Design review of the part built by this model. Coordinates are the model's own, in mm. Face numbers are marked on the shaded views. A direction names the side the tool comes from. Give positions to 0.01 mm unless a question says otherwise; leave off trailing zeros. Order: outer loops, then holes, each group sorted by start corner. A loop starts at its lowest first (then second) coordinate and runs counter-clockwise, first axis right, second up. Notation, with made-up numbers: (55, -25) -> (65, -25) arc R28 cw to (65, -6) -> close; hole circle Ø7 at (46, 52.25). An arc over 180 degrees is marked (long way). Return JSON: item names as keys, results as strings.
```python
from build123d import *

# Parameters (mm, degrees)
SKETCH1_R           = 11.1125
BOSS_EXTRUDE1_DEPTH = 29.028571429
SKETCH2_R           = 9.525
BOSS_EXTRUDE2_DEPTH = 44.45
SKETCH3_W           = 2.553411187
SKETCH3_H           = 10.53028371
SKETCH3_W_2         = 2.754606744
CUT_EXTRUDE1_DEPTH  = 44.45
SKETCH4_R           = 6.35
BOSS_EXTRUDE3_DEPTH = 1.5875
SKETCH5_W           = 1.859243387
SKETCH5_H           = 6.148361062
SKETCH5_W_2         = 2.232892279
CUT_EXTRUDE2_DEPTH  = 1.5875
SKETCH6_R           = 2.38125
BOSS_EXTRUDE4_DEPTH = 11.1125


with BuildPart() as part:
    # Sketch1 → Boss-Extrude1 (new body)
    with BuildSketch(Plane(origin=(0, 0, 0), x_dir=(0, 0, -1), z_dir=(1, 0, 0))):
        Circle(SKETCH1_R)
    extrude(amount=BOSS_EXTRUDE1_DEPTH)

    # Sketch2 → Boss-Extrude2 (add)
    with BuildSketch(Plane(origin=(29.028571429, 0, 0), x_dir=(0, 0, -1), z_dir=(1, 0, 0))):
        Circle(SKETCH2_R)
    extrude(amount=BOSS_EXTRUDE2_DEPTH)

    # Sketch3 → Cut-Extrude1 (cut)
    with BuildSketch(Plane(origin=(73.478571429, 0, 0), x_dir=(0, 0, -1), z_dir=(1, 0, 0))):
        with Locations((-9.214205594, 0)):
            Rectangle(SKETCH3_W, SKETCH3_H)
        with Locations((9.314803372, 0)):
            Rectangle(SKETCH3_W_2, SKETCH3_H)
    extrude(amount=-CUT_EXTRUDE1_DEPTH, mode=Mode.SUBTRACT)

    # Sketch4 → Boss-Extrude3 (add)
    with BuildSketch(Plane.ZY):
        Circle(SKETCH4_R)
    extrude(amount=BOSS_EXTRUDE3_DEPTH)

    # Sketch5 → Cut-Extrude2 (cut)
    with BuildSketch(Plane.ZY.offset(1.5875)):
        with Locations((-6.485871694, 0)):
            Rectangle(SKETCH5_W, SKETCH5_H)
        with Locations((6.67269614, 0)):
            Rectangle(SKETCH5_W_2, SKETCH5_H)
    extrude(amount=-CUT_EXTRUDE2_DEPTH, mode=Mode.SUBTRACT)

    # Sketch6 → Boss-Extrude4 (add)
    with BuildSketch(Plane.ZY.offset(1.5875)):
        Circle(SKETCH6_R)
    extrude(amount=BOSS_EXTRUDE4_DEPTH)


solid = part.part
```
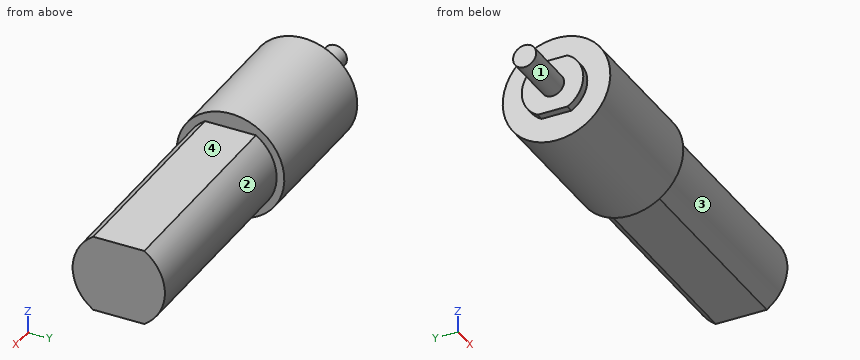
Item 1: Machinability: for the marked faces 1, 2, 3 and 4, which of the approach directions +Z, -Z, +X, -X, +Y, -Y give a long, thin tool a straight path to every point of the face, cutting with its end or side? Answer none if there is none.
Result set:
{"face 1": "-X", "face 2": "+X, +Y", "face 3": "+X, -Y", "face 4": "+Z, +X, +Y, -Y"}
Item 2: Add section D-D (y = -7.75). Give the boundary of the cut face in (x, z).
Result set:
{"outline": "(0, -7.96) -> (29.03, -7.96) -> (29.03, -5.54) -> (73.48, -5.54) -> (73.48, 5.54) -> (29.03, 5.54) -> (29.03, 7.96) -> (0, 7.96) -> close"}
Item 3: For pin 1 (1.5 mm diameter, centred on x = 22, z = 1, fed in from -Y); pin 2 (8 mm diameter, centred on x = 16.5, z = -7, fed in from +Y); pin 3 (12 mm diameter, centred on x = 55.5, y = 0.5, fed in from -Z); pin 4 (10 mm diameter, centred on y = -5, z = 3, fed in from -X), all flat-tipped, find the tip position at first contact; note any pin that passes through.
Result set:
{"pin 1": "stops at y = -11.11", "pin 2": "stops at y = 10.7", "pin 3": "stops at z = -7.94", "pin 4": "stops at x = -12.7"}
Item 4: Wall thickness on L1, parallel to Z at x = 67, y = 4; L2, parallel to X at y = 9.25, z = -1.5; L3, parallel to X at y = 1.5, z = -8.25: over which ranges is each line inside the solid? List them lowest first. Write a range as [from, to].
Result set:
{"L1": "z = [-7.94, 7.94]", "L2": "x = [0, 73.48]", "L3": "x = [0, 29.03]"}
Item 5: Add section C-C (x = -3). Give the boundary of the cut face in (y, z).
Result set:
{"outline": "circle Ø4.76 at (0, 0)"}
Item 6: Add section A-A (y = 0). Give the boundary of the cut face in (x, z).
Result set:
{"outline": "(-12.7, -2.38) -> (-1.59, -2.38) -> (-1.59, -5.56) -> (0, -5.56) -> (0, -11.11) -> (29.03, -11.11) -> (29.03, -7.94) -> (73.48, -7.94) -> (73.48, 7.94) -> (29.03, 7.94) -> (29.03, 11.11) -> (0, 11.11) -> (0, 5.56) -> (-1.59, 5.56) -> (-1.59, 2.38) -> (-12.7, 2.38) -> close"}
